Part print with two shaded views. Sizes in mm from the minimum x, y, z corner. A direction names the side the tool comes from. Coordinates: 2 decimals unless noted, no trailing zeros. Loops run counter-clockwise (first coordinate to the right, second up) from the corner with the lowest first, then second, coordinate; pieces in that order, holes last. Notation, with made-up numbers: (3, -26) -> (17, -26) arc R27 cw to (17, 10) -> close; hole circle Ø11 at (23.5, 49). An arc over 180 degrees is marked (long way). Use one line per item in the form item = value.
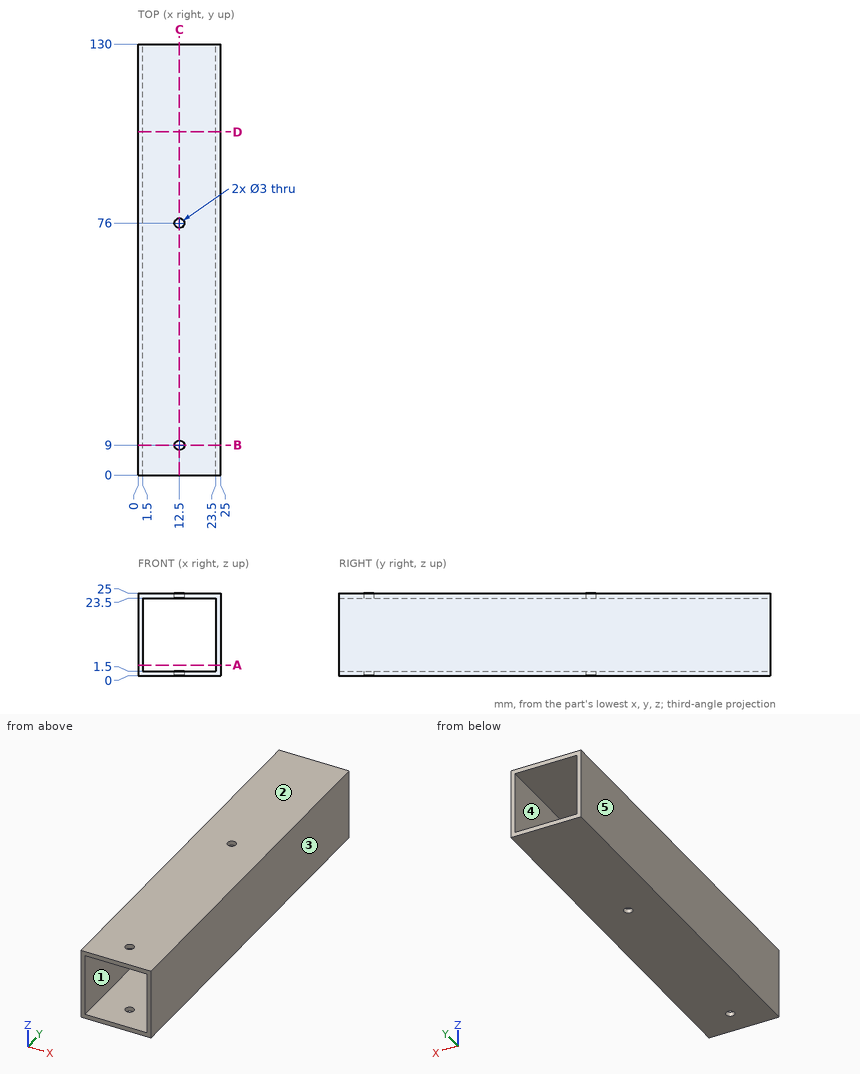
Q1. Which spindle directions (+Z, -Z, +X, -X, +Y, -Y) get a long thin tool onto all of the face, cutting with end or side? Do the marked faces 4 and 5. Say none if no direction does.
Result:
face_4 = +Y, -Y
face_5 = +Z, -Z, -X, +Y, -Y
Q2. Wall check: line 1 along Y through (x, z) = (12.5, 1.15); line 2 along Z through (x, y) = (4.5, 81.5); line 3 along X through (y, z) = (9, 0.55). Give the ranges that are in metal, low to high.
Result:
line_1 = 0 to 7.5, 10.5 to 74.5, 77.5 to 130
line_2 = 0 to 1.5, 23.5 to 25
line_3 = 0 to 11, 14 to 25
Q3. Mould opens along Z. For the marked faces 1, 2 and 3 say: released by +Z, released by -Z, zero draft, split by the parting line, or undercut.
Result:
face_1 = undercut
face_2 = released by +Z
face_3 = zero draft
Q4. Band-saw the part on A-A, the plane z = 3.25. Write the cut outline in (x, y), and give its area (3 significant figures).
Result:
outline = (0, 0) -> (1.5, 0) -> (1.5, 130) -> (0, 130) -> close; (23.5, 0) -> (25, 0) -> (25, 130) -> (23.5, 130) -> close
area = 390 mm2
Q5. Pin check, flat tip, straight feed: pin 1 Ø1.8 at (x, y) = (12.5, 9) entering from -Z. Stop position of the tip, or through.
Result:
pin_1 = through
Q6. Band-saw the part on C-C, the plane x = 12.5. Write the cut outline in (y, z), and give its area (3 significant figures).
Result:
outline = (0, 0) -> (7.5, 0) -> (7.5, 1.5) -> (0, 1.5) -> close; (0, 23.5) -> (7.5, 23.5) -> (7.5, 25) -> (0, 25) -> close; (10.5, 0) -> (74.5, 0) -> (74.5, 1.5) -> (10.5, 1.5) -> close; (10.5, 23.5) -> (74.5, 23.5) -> (74.5, 25) -> (10.5, 25) -> close; (77.5, 0) -> (130, 0) -> (130, 1.5) -> (77.5, 1.5) -> close; (77.5, 23.5) -> (130, 23.5) -> (130, 25) -> (77.5, 25) -> close
area = 372 mm2
Q7. Band-saw the part on B-B, the plane y = 9. Write the cut outline in (x, z).
Result:
outline = (0, 0) -> (11, 0) -> (11, 1.5) -> (1.5, 1.5) -> (1.5, 23.5) -> (11, 23.5) -> (11, 25) -> (0, 25) -> close; (14, 0) -> (25, 0) -> (25, 25) -> (14, 25) -> (14, 23.5) -> (23.5, 23.5) -> (23.5, 1.5) -> (14, 1.5) -> close
Q8. Band-saw the part on D-D, the plane y = 103.5. Write the cut outline in (x, z), and give its area (3 significant figures).
Result:
outline = (0, 0) -> (25, 0) -> (25, 25) -> (0, 25) -> close; hole (1.5, 1.5) -> (23.5, 1.5) -> (23.5, 23.5) -> (1.5, 23.5) -> close
area = 141 mm2
